Input: part model. Units: mm. Frame: model coordinates. A direction names the side the tool comes from. Give positions to 0.01 mm unless a question says otherwise; leave off trailing zeros. Write each loop counter-clockwise with the first axis right and the second up, starting at its lowest first coordinate (ties: lowest second). Pieces come first, ordered by that corner, then holes. Notation, with made-up numbers: M 48.5,32.25 L 60.5,32.25 A11 cw 60.5,44.25 Z; hole C 61,44.25 d1. An arc over 180 degrees is marked long. Use CSV: the item, a comma, the result in double quotes. Start each with the question number.
from build123d import *

# Parameters (mm, degrees)
SCHIZZO1_R                                           = 100
SCHIZZO1_R_2                                         = 32
SCHIZZO1_R_3                                         = 5
ESTRUSIONE1_DEPTH                                    = 12
SMUSSO1_SIZE                                         = 1
M10_FORO_LAMATO_PER_VITE_A_TESTA_ESAGONA_D           = 11
M10_FORO_LAMATO_PER_VITE_A_TESTA_ESAGONA_CBORE_D     = 21.475
M10_FORO_LAMATO_PER_VITE_A_TESTA_ESAGONA_CBORE_DEPTH = 9


with BuildPart() as part:
    # Schizzo1 → Estrusione1 (new body)
    with BuildSketch(Plane.XY):
        Circle(SCHIZZO1_R)
        Circle(SCHIZZO1_R_2, mode=Mode.SUBTRACT)
        with Locations((-73.612159322, 42.5)):
            Circle(SCHIZZO1_R_3, mode=Mode.SUBTRACT)
        with Locations((73.612159322, 42.5)):
            Circle(SCHIZZO1_R_3, mode=Mode.SUBTRACT)
        with Locations((0, -85)):
            Circle(SCHIZZO1_R_3, mode=Mode.SUBTRACT)
    extrude(amount=ESTRUSIONE1_DEPTH)

    # Smusso1
    smusso1_edges = [part.edges().sort_by_distance(p)[0] for p in [
        (68.612159322, 42.5, 0),
        (-5, -85, 0),
        (-100, 0, 0),
        (-32, 0, 0),
        (-78.612159322, 42.5, 0),
    ]]
    chamfer(smusso1_edges, length=SMUSSO1_SIZE)

    # M10 Foro lamato per vite a testa esagonale (parzialmente filettata)2 (through all)
    with Locations(Plane(origin=(-8.776237921, -26.129151675, 12), x_dir=(0.9999999999963068, -2.7178071316053742e-06, 0), z_dir=(0, 0, 1))):
        with Locations((-60.505865396, 66.129175527), (8.776166907, -53.870824473), (78.05819921, 66.129175527)):
            CounterBoreHole(M10_FORO_LAMATO_PER_VITE_A_TESTA_ESAGONA_D / 2, M10_FORO_LAMATO_PER_VITE_A_TESTA_ESAGONA_CBORE_D / 2, M10_FORO_LAMATO_PER_VITE_A_TESTA_ESAGONA_CBORE_DEPTH)


solid = part.part
Q1. Set-up query: faces 4 (the flat face through (64, 43, 3)), 5 (the cylindrical face through (-0.166, -74.503, 1.479)). Return all of +Z, -Z, +X, -X, +Y, -Y with unobstructed straight access to the full face (end or side cutting, diameter ignored); none if empty.
Q2. Material intervals for L1, parallel to Y at x = 0, z = 5; L2, parallel to Y at x = 0, z = 2.45; L3, parallel to X at y = 42.5, z = 2, sorted ascending. Write a range as [from, to].
Q3. Pull-direction query (X, two-part tool) for faces 1 (the flat face through (43, 1, 0)), 2 (the cylindrical face through (95.38, 30.04, 6.42)), 3 (the flat face through (-3, -75, 3)); classes: released by +X, released by -X, zero draft, split by the parting line, or undercut.
Q4. Section B-B, the plane x = 0. Return the cut outline in (y, z), and give its area (3 significant figures).
Q5. Section D-D, the plane y = 42.5. Give the number of separate pieces and of enclosed holes in the cut face, and give its area (3 significant figures).
Q6. Section A-A, the plane y = 0. Return the cut outline in (x, z), and give its area (3 significant figures).
Q7. Section C-C, the plane z = 7.5. Return the cut outline in (x, y) (1 decimal), and give its area (3 significant figures).
Q8. First-contact query: pin 1 Ø13 at (x, y) = (-69.28, 40) entering from +Z; pin 2 Ø5 at (x, z) = (-49.5, 6.5) entering from +Y; pin 3 Ø4 at (y, z) = (11.5, 2) entering from +X. Flat tips, straight axial feed; report the tip coordinate or a pass-through.
Check result:
1,face 4,"+Z"
1,face 5,"+Z, -Z"
2,L1,"y = [-100, -90.74], [-69.26, -32], [32, 100]"
2,L2,"y = [-100, -90], [-74.5, -32], [32, 100]"
2,L3,"x = [-90.52, -78.61], [-64.38, 64.38], [78.61, 90.52]"
3,face 1,"zero draft"
3,face 2,"split by the parting line"
3,face 3,"undercut"
4,outline,"M -100,1 L -99,0 L -91,0 L -90,1 L -90,3 L -90.74,3 L -90.74,12 L -100,12 Z; M -74.5,0 L -33,0 L -32,1 L -32,12 L -69.26,12 L -69.26,3 L -74.5,3 Z; M 32,1 L 33,0 L 99,0 L 100,1 L 100,12 L 32,12 Z"
4,area,"1,390 mm²"
5,separate pieces,"3"
5,enclosed holes,"0"
5,area,"1,710 mm²"
6,outline,"M -100,1 L -99,0 L -33,0 L -32,1 L -32,12 L -100,12 Z; M 32,1 L 33,0 L 99,0 L 100,1 L 100,12 L 32,12 Z"
6,area,"1,630 mm²"
7,outline,"C 0,0 d200; hole C -69.3,40 d21.5; hole C 0,0 d64; hole C 0,-80 d21.5; hole C 69.3,40 d21.5"
7,area,"27,100 mm²"
8,pin 1,"stops at z = 3"
8,pin 2,"stops at y = 88.27"
8,pin 3,"stops at x = 99.55"
